The listing builds one solid part. Answer for the finished solid, in the listing's coordinates (mm). A direction names the side the tool comes from. Give positions to 0.01 mm unless a question says otherwise; leave off trailing zeros. Write each loop counter-clockwise with the first axis right and the second up, starting at its lowest first coordinate (ties: lowest second). Pieces come first, ordered by that corner, then holes. Notation, with made-up numbers: (21.5, 2.5) - (62.5, 2.5) arc R24 ccw to (62.5, 32.5) - close; hole circle Ø5 at (16.5, 32). An arc over 180 degrees is marked (long way). Answer as CSV lines item,"result". Start each with the question number.
(1) Each of these flat-tipped pins is pushed along its axis until it touches: pin 1 Ø12.5 at (y, z) = (12.5, 30) entering from +X; pin 2 Ø3.5 at (x, z) = (-10, 16.5) entering from +Y; pin 3 Ø2.5 at (x, y) = (16.5, 6) entering from -Z. Where does it stop, or does it pass through?
(2) For a pull along X with two mould halves and no side action, classify faces 4 (the face through (-15.9, 25, -32)), 5 (the face through (-14.05, 17, -32)), 6 (the face through (-22, 14, -24.2)), 7 (the face through (-22, 18.056, 32)) as pulls with the +X half, pulls with the -X half, needs draft (parallel to the pull), parting line crosses it, or undercut.
(3) Find section C-C (x = -25.5). Write down the section's boundary in (y, z).
(4) Find section A-A (y = 13.5). Write down the section's boundary in (x, z).
(5) Find section B-B (y = 24). Write down the section's boundary in (x, z), then the cut area to 3 significant figures.
(6) Find section D-D (z = -33). Write down the section's boundary in (x, y) (3 decimals), then the cut area to 3 significant figures.
(7) For faces 1 (the face through (-11, 7, 14.5)), 2 (the face through (-11, 7, 17.5)), 3 (the face through (-28.15, 24, 32)), determine the directions among +Z, -Z, +X, -X, +Y, -Y from which every point of the face is accessible in a straight line to the end or side of a thin tool.
(8) Straight lines are drawn through the part: probe 1 along Z at (x, y) = (-15.5, 21); probe 2 along Y at (x, z) = (18, 19); probe 3 along Z at (x, y) = (15, 8.5). For each, find the intervals that lie inside material, in ascending order.
from build123d import *

# Parameters (mm, degrees)
SKETCH1_W           = 60
SKETCH1_H           = 80
BOSS_EXTRUDE1_DEPTH = 3
BOSS_EXTRUDE2_START = 40
SKETCH3_W           = 12.25
SKETCH3_H           = 15.056176196
SKETCH3_R           = 0.5
SKETCH3_W_2         = 1.85
SKETCH3_H_2         = 28
BOSS_EXTRUDE2_DEPTH = 15.8
BOSS_EXTRUDE3_START = -40
SKETCH3_3_W         = 12.25
SKETCH3_3_H         = 15.056176196
SKETCH3_3_R         = 0.5
SKETCH3_3_W_2       = 1.85
SKETCH3_3_H_2       = 28
BOSS_EXTRUDE3_DEPTH = 15.8
BOSS_EXTRUDE4_START = 14.5
SKETCH4_W           = 5
SKETCH4_H           = 8
SKETCH4_R           = 0.5
BOSS_EXTRUDE4_DEPTH = 3


with BuildPart() as part:
    # Sketch1 → Boss-Extrude1 (new body)
    with BuildSketch(Plane(origin=(0, 0, 0), x_dir=(1, 0, 0), z_dir=(0, 1, 0))):
        Rectangle(SKETCH1_W, SKETCH1_H)
    extrude(amount=BOSS_EXTRUDE1_DEPTH)

    # Sketch3 → Boss-Extrude2 (add)
    with BuildSketch(Plane.XY.offset(BOSS_EXTRUDE2_START)):
        Polygon((-15.9, 18.056176196), (-15.9, 3), (-14.05, 3), (-14.05, 31), (-15.9, 31), align=None)
        with Locations((-22.025, 10.528088098)):
            Rectangle(SKETCH3_W, SKETCH3_H)
        with Locations((-22.025, 16.056176196)):
            Circle(SKETCH3_R, mode=Mode.SUBTRACT)
        with Locations((-29.075, 17)):
            Rectangle(SKETCH3_W_2, SKETCH3_H_2)
    extrude(amount=-BOSS_EXTRUDE2_DEPTH)

    # Sketch3<3> → Boss-Extrude3 (add)
    with BuildSketch(Plane.XY.offset(BOSS_EXTRUDE3_START)):
        Polygon((-15.9, 18.056176196), (-15.9, 3), (-14.05, 3), (-14.05, 31), (-15.9, 31), align=None)
        with Locations((-22.025, 10.528088098)):
            Rectangle(SKETCH3_3_W, SKETCH3_3_H)
        with Locations((-22.025, 16.056176196)):
            Circle(SKETCH3_3_R, mode=Mode.SUBTRACT)
        with Locations((-29.075, 17)):
            Rectangle(SKETCH3_3_W_2, SKETCH3_3_H_2)
    extrude(amount=BOSS_EXTRUDE3_DEPTH)

    # Sketch4 → Boss-Extrude4 (add)
    with BuildSketch(Plane.XY.offset(BOSS_EXTRUDE4_START)):
        with Locations((16.5, 7)):
            Rectangle(SKETCH4_W, SKETCH4_H)
        with Locations((16.5, 8.9)):
            Circle(SKETCH4_R, mode=Mode.SUBTRACT)
        with Locations((-11.05, 7)):
            Rectangle(SKETCH4_W, SKETCH4_H)
        with Locations((-11.05, 8.9)):
            Circle(SKETCH4_R, mode=Mode.SUBTRACT)
    extrude(amount=BOSS_EXTRUDE4_DEPTH)


solid = part.part
Result set:
1,pin 1,"x = -14.05"
1,pin 2,"y = 11"
1,pin 3,"z = 14.5"
2,face 4,"undercut"
2,face 5,"pulls with the +X half"
2,face 6,"needs draft"
2,face 7,"undercut"
3,outline,"(0, -40) - (18.06, -40) - (18.06, -24.2) - (3, -24.2) - (3, 24.2) - (18.06, 24.2) - (18.06, 40) - (0, 40) - close"
4,outline,"(-30, -40) - (-14.05, -40) - (-14.05, -24.2) - (-30, -24.2) - close; (-30, 24.2) - (-14.05, 24.2) - (-14.05, 40) - (-30, 40) - close"
5,outline,"(-30, -40) - (-28.15, -40) - (-28.15, -24.2) - (-30, -24.2) - close; (-30, 24.2) - (-28.15, 24.2) - (-28.15, 40) - (-30, 40) - close; (-15.9, -40) - (-14.05, -40) - (-14.05, -24.2) - (-15.9, -24.2) - close; (-15.9, 24.2) - (-14.05, 24.2) - (-14.05, 40) - (-15.9, 40) - close"
5,area,"117 mm^2"
6,outline,"(-30, 0) - (30, 0) - (30, 3) - (-14.05, 3) - (-14.05, 31) - (-15.9, 31) - (-15.9, 18.056) - (-28.15, 18.056) - (-28.15, 31) - (-30, 31) - close; hole circle Ø1 at (-22.025, 16.056)"
6,area,"467 mm^2"
7,face 1,"-Z, +X, -X, +Y"
7,face 2,"+Z, +X, -X, +Y"
7,face 3,"+Z, -Z, +Y"
8,probe 1,"-40 to -24.2, 24.2 to 40"
8,probe 2,"0 to 3"
8,probe 3,"14.5 to 17.5"
